The model under review builds one solid part; all positions refer to its coordinate system, in mm. A direction names the side the tool comes from. Round coordinates to 2 decimals unless told otherwise and drop trailing zeros. Order: outer loops, then holes, each group sorted by start corner. A loop starts at its lowest first (then second) coordinate and runs counter-clockwise, first axis right, second up.
from build123d import *

# Parameters (mm, degrees)
BOSS_EXTRUDE1_DEPTH      = 5
BOSS_EXTRUDE4_DEPTH      = 30
BOSS_EXTRUDE4_DEPTH_BACK = 35
SKETCH5_W                = 42.3
SKETCH5_H                = 5
CUT_EXTRUDE5_DEPTH       = 10
SKETCH9_W                = 14
SKETCH9_H                = 5
BOSS_EXTRUDE5_DEPTH      = 35
FILLET1_R                = 10
BOSS_EXTRUDE6_DEPTH      = 4
BOSS_EXTRUDE7_DEPTH      = 4
SKETCH12_R               = 2.5
CUT_EXTRUDE6_DEPTH       = 79.277111821
BOSS_EXTRUDE8_DEPTH      = 5
FILLET2_R                = 20


with BuildPart() as part:
    # Sketch1 → Boss-Extrude1 (new body)
    with BuildSketch(Plane(origin=(0, 0, 0), x_dir=(1, 0, 0), z_dir=(0, 1, 0))):
        Polygon((-10.255294708, 42.808405172), (11.744705292, 42.808405172), (21.894705292, 42.808405172), (21.894705292, 3.008405172), (21.894705292, -4.991594828), (-20.405294708, -4.991594828), (-20.405294708, 3.008405172), (-20.405294708, 42.808405172), align=None)
    extrude(amount=BOSS_EXTRUDE1_DEPTH)

    # Sketch5 → Boss-Extrude4 (add, two sides: drawn at the far end of the back side and taken through both)
    with BuildSketch(Plane(origin=(0, 5, 0), x_dir=(1, 0, 0), z_dir=(0, 1, 0)).offset(-BOSS_EXTRUDE4_DEPTH_BACK)):
        with Locations((0.744705292, 40.308405172)):
            Rectangle(SKETCH5_W, SKETCH5_H)
    extrude(amount=BOSS_EXTRUDE4_DEPTH + BOSS_EXTRUDE4_DEPTH_BACK)

    # Sketch8 → Cut-Extrude5 (cut)
    with BuildSketch(Plane.XY.offset(-37.808405172)):
        with BuildLine():
            Line((-7.5, 22), (7.5, 22))
            ThreePointArc((7.5, 22), (11, 18.5), (7.5, 15))
            Line((7.5, 15), (-7.5, 15))
            ThreePointArc((-7.5, 15), (-11, 18.5), (-7.5, 22))
        make_face()
        with BuildLine():
            Line((-7.5, -10), (7.5, -10))
            ThreePointArc((7.5, -10), (11, -13.5), (7.5, -17))
            Line((7.5, -17), (-7.5, -17))
            ThreePointArc((-7.5, -17), (-11, -13.5), (-7.5, -10))
        make_face()
    extrude(amount=-CUT_EXTRUDE5_DEPTH, mode=Mode.SUBTRACT)

    # Sketch9 → Boss-Extrude5 (add)
    with BuildSketch(Plane.ZY.offset(20.405294708)):
        with Locations((-2.008405172, 2.5)):
            Rectangle(SKETCH9_W, SKETCH9_H)
    extrude(amount=BOSS_EXTRUDE5_DEPTH)

    # Fillet1
    fillet1_edges = [part.edges().sort_by_distance(p)[0] for p in [
        (-55.405294708, 2.5, 4.991594828),
    ]]
    fillet(fillet1_edges, radius=FILLET1_R)

    # Sketch10 → Boss-Extrude6 (add)
    with BuildSketch(Plane.ZY.offset(20.405294708)):
        Polygon((-42.808405172, 2.5), (-42.808405172, 22.5), (-9.008405172, 2.5), (-42.808405172, -17.5), align=None)
    extrude(amount=-BOSS_EXTRUDE6_DEPTH)

    # Sketch11 → Boss-Extrude7 (add)
    with BuildSketch(Plane(origin=(21.894705292, 0, 0), x_dir=(0, 0, -1), z_dir=(1, 0, 0))):
        Polygon((37.808405172, 19.541420118), (37.808405172, -14.541420118), (13.233405172, 0), (13.233405172, 5), align=None)
    extrude(amount=-BOSS_EXTRUDE7_DEPTH)

    # Sketch12 → Cut-Extrude6 (cut, through all)
    with BuildSketch(Plane(origin=(0, 5, 0), x_dir=(1, 0, 0), z_dir=(0, 1, 0))):
        with Locations(Location((-47.405294708, 3.008405172, 0), (0, 0, 270))):
            Circle(SKETCH12_R)
    extrude(amount=-CUT_EXTRUDE6_DEPTH, mode=Mode.SUBTRACT)

    # Sketch13 → Boss-Extrude8 (add)
    with BuildSketch(Plane.XZ):
        Polygon((-40.733122826, -9.008405172), (-20.405294708, -34.32558847), (-20.405294708, -9.008405172), align=None)
    extrude(amount=-BOSS_EXTRUDE8_DEPTH)

    # Fillet2
    fillet2_edges = [part.edges().sort_by_distance(p)[0] for p in [
        (21.894705292, 2.5, 4.991594828),
    ]]
    fillet(fillet2_edges, radius=FILLET2_R)


solid = part.part
(1) We need section C-C (y = 1.5). Give the boundary of the cut face in (x, z), and give its area (3 significant figures).
(2) The part is to be moulded in two halves that separate along X. For faces 1 (the flat face through (19.92, 12.17, -25.35)), 2 (the flat face through (-20.405, 5, -35)), 3 (the flat face through (0, -17, -40)), 4 (the cylindrical face through (11, -13.4, -40.3)), say which applies: pulls with the +X half, pulls with the -X half, needs draft (parallel to the pull), parting line crosses it, or undercut.
(3) To check wall thickness, follow L1, parallel to X at y = -9, z = -28.5; L2, parallel to Y at x = -12.5, z = -32.5; L3, parallel to Z at x = -9, y = 26. State the ranges of each line that lie inside material, in increasing order.
(4) Tool access review of faces 5 (the flat face through (-16.405, -4, -31)), 6 (the flat face through (0, -30, -40)), 7 (the flat face through (0, 15, -40)), 8 (the flat face through (-30.71, 2.46, -21.49)), 9 (the flat face through (-9, 5, -11)): name each direction out of +Z, -Z, +X, -X, +Y, -Y from which nothing blocks a thin tool from reaching the whole face with its end or side.
(5) Clearance check with flat-ended pins moving along their axes: P1, Ø2.5, axis at x = -44.5, y = 3, coming from the -Z side; P2, Ø1, axis at x = -17, z = -9.5, coming from the +Y side; P3, Ø1.5, axis at y = -0.5, z = -7, coming from the -X side; P4, Ø15, axis at x = 11, y = -21, coming from the +Z side. State where each tip first meets the part, or that it passes through.
(6) We need section D-D (x = 10). Give the boundary of the cut face in (y, z), and give its area (3 significant figures).
(7) We need section A-A (x = -19). Give the boundary of the cut face in (y, z).
(8) We need section B-B (z = -39). Give the boundary of the cut face in (x, y).
Verdict:
1. outline: (-55.41, -9.01) - (-40.73, -9.01) - (-20.41, -34.33) - (-20.41, -42.81) - (21.89, -42.81) - (21.89, -15.01) arc R20 ccw to (1.89, 4.99) - (-45.41, 4.99) arc R10 ccw to (-55.41, -5.01) - close; hole circle Ø5 at (-47.41, -3.01)
1. area: 2,640 mm2
2. face 1: needs draft
2. face 2: pulls with the -X half
2. face 3: undercut
2. face 4: undercut
3. L1: x = -20.41 to -16.41, 17.89 to 21.89
3. L2: y = 0 to 5
3. L3: z = -42.81 to -37.81
4. face 5: +Z, -Y
4. face 6: +Z, -Z, +X, -X, -Y
4. face 7: +Z, -Z
4. face 8: -Z, -X, +Y, -Y
4. face 9: +Z, +Y
5. P1: stops at z = -9.01
5. P2: stops at y = 5
5. P3: stops at x = -55.41
5. P4: stops at z = -37.81
6. outline: (-30, -42.81) - (-15.95, -42.81) - (-15.95, -37.81) - (-30, -37.81) - close; (-11.05, -42.81) - (16.05, -42.81) - (16.05, -37.81) - (5, -37.81) - (5, 3.28) - (0, 3.28) - (0, -37.81) - (-11.05, -37.81) - close; (20.95, -42.81) - (35, -42.81) - (35, -37.81) - (20.95, -37.81) - close
6. area: 481 mm2
7. outline: (-30, -42.81) - (35, -42.81) - (35, -37.81) - (19.54, -37.81) - (5, -13.23) - (5, 4.99) - (0, 4.99) - (0, -13.23) - (-14.54, -37.81) - (-30, -37.81) - close
8. outline: (-20.41, -30) - (21.89, -30) - (21.89, 35) - (-20.41, 35) - close; hole (-7.5, -17) - (7.5, -17) arc R3.5 ccw to (7.5, -10) - (-7.5, -10) arc R3.5 ccw to start; hole (-7.5, 15) - (7.5, 15) arc R3.5 ccw to (7.5, 22) - (-7.5, 22) arc R3.5 ccw to start
